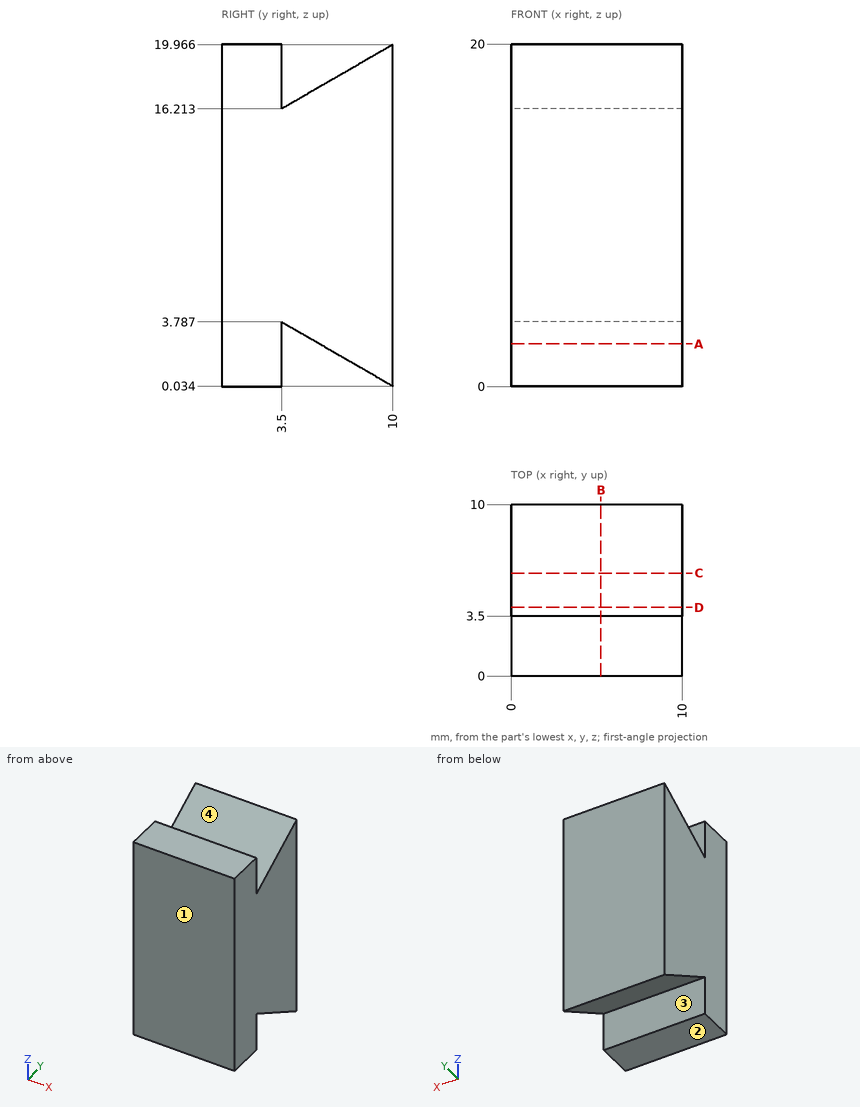
The drawing under review shows one solid part. Ordinate dimensions are in mm from its lowest x, y, z. Give positions to 0.01 mm unless a question says otherwise; leave off trailing zeros. Order: outer loops, then holes, each group sorted by start corner. A loop starts at its lowest first (then second) coordinate and runs counter-clockwise, first axis right, second up. Notation, with made-up numbers: (-25, 32) -> (-6, 32) arc R9 cw to (-6, 49) -> close; hole circle Ø2 at (-1, 1). An arc over 180 degrees is marked (long way). Write item = value, one per line. Start each with the question number.
(1) We need section C-C on y = 6. Write out the cut boundary in (x, z).
(2) To check wall thickness, follow line 1 along Y through (x, z) = (9, 3.25); line 2 along Y through (x, z) = (7.25, 17.5); line 3 along Z through (x, y) = (3.75, 5.25). State the ranges of each line that lie inside material, in increasing order.
(3) We need section B-B on x = 5.25. Write out the cut boundary in (y, z), plus the area to 3 significant figures.
(4) For pin 1 (5 mm diameter, centred on x = 2.5, y = 7, fed in from +Z), flat-tipped, find the tip position at first contact; note if it passes through.
(5) Mouldability with a two-part tool opening along Y and no side actions: class the marked faces 1, 2, 3 and 4 as +Y half, -Y half, draft (parallel to the pull), parting line (faces both ways), or undercut.
(6) We need section A-A on z = 2.5. Write out the cut boundary in (x, y), plus the area to 3 significant figures.
(7) We need section D-D on y = 4. Write out the cut boundary in (x, z), plus the area to 3 significant figures.
Numbers:
q1.outline = (0, 2.34) -> (10, 2.34) -> (10, 17.66) -> (0, 17.66) -> close
q2.line_1 = 0 to 3.5, 4.43 to 10
q2.line_2 = 0 to 3.5, 5.73 to 10
q2.line_3 = 2.78 to 17.22
q3.outline = (0, 0) -> (3.5, 0) -> (3.5, 3.79) -> (10, 0.03) -> (10, 19.97) -> (3.5, 16.21) -> (3.5, 20) -> (0, 20) -> close
q3.area = 175 mm^2
q4.pin_1 = 19.68
q5.face_1 = -Y half
q5.face_2 = draft
q5.face_3 = undercut
q5.face_4 = undercut
q6.outline = (0, 0) -> (10, 0) -> (10, 3.5) -> (0, 3.5) -> close; (0, 5.73) -> (10, 5.73) -> (10, 10) -> (0, 10) -> close
q6.area = 77.7 mm^2
q7.outline = (0, 3.5) -> (10, 3.5) -> (10, 16.5) -> (0, 16.5) -> close
q7.area = 130 mm^2
